```python
from build123d import *

# Parameters (mm, degrees)
PROFILE_W               = 12.7
PROFILE_H               = 22.86
PROFILE_W_2             = 6.35
PROFILE_H_2             = 12.7
BOSS_EXTRUDE1_DEPTH     = 12.7
SCREWHOLE_R             = 2.159
CUT_EXTRUDE1_DEPTH      = 7.35
CUT_EXTRUDE1_DEPTH_BACK = 7.35
SKETCH3_R               = 3.683
SKETCH3_R_2             = 2.159
CUT_EXTRUDE2_DEPTH      = 4.064
BOSS_EXTRUDE2_DEPTH     = 35.56


with BuildPart() as part:
    # Profile → Boss-Extrude1 (new body, symmetric)
    with BuildSketch(Plane.XY):
        with Locations((0, 11.43)):
            Rectangle(PROFILE_W, PROFILE_H)
        with Locations((3.175, -6.35)):
            Rectangle(PROFILE_W_2, PROFILE_H_2)
    extrude(amount=BOSS_EXTRUDE1_DEPTH, both=True)

    # ScrewHole → Cut-Extrude1 (cut, two sides)
    with BuildSketch(Plane.ZY) as cut_extrude1_sk:
        with Locations((0, -6.35)):
            Circle(SCREWHOLE_R)
    extrude(amount=CUT_EXTRUDE1_DEPTH, mode=Mode.SUBTRACT)
    extrude(cut_extrude1_sk.sketch, amount=-CUT_EXTRUDE1_DEPTH_BACK, mode=Mode.SUBTRACT)

    # Sketch3 → Cut-Extrude2 (cut)
    with BuildSketch(Plane(origin=(6.35, 0, 0), x_dir=(0, 0, -1), z_dir=(1, 0, 0))):
        with Locations((0, -6.35)):
            Circle(SKETCH3_R)
        with Locations((0, -6.35)):
            Circle(SKETCH3_R_2, mode=Mode.SUBTRACT)
    extrude(amount=-CUT_EXTRUDE2_DEPTH, mode=Mode.SUBTRACT)

    # Sketch5 → Boss-Extrude2 (add)
    with BuildSketch(Plane.XZ.offset(12.7)):
        with BuildLine():
            Line((-1.27, -57.15), (3.81, -57.15))
            Line((3.81, -57.15), (1.016473553, -32.70664359))
            ThreePointArc((1.016473553, -32.70664359), (2.103447964, -24.502378011), (6.930571429, -17.78))
            Line((6.930571429, -17.78), (6.35, -12.7))
            Line((6.35, -12.7), (0, -12.7))
            Line((0, -12.7), (-6.35, -12.7))
            Line((-6.35, -12.7), (-1.27, -57.15))
        make_face()
    extrude(amount=-BOSS_EXTRUDE2_DEPTH)


solid = part.part
```
The listing builds one solid part. Answer for the finished solid, in the listing's coordinates (mm). A direction names the side the tool comes from. Round coordinates to 2 decimals unless told otherwise and drop trailing zeros. Loops run counter-clockwise (first coordinate to the right, second up) from the corner with the lowest first, then second, coordinate; pieces in that order, holes last. Notation, with made-up numbers: (58.5, 86) - (85.5, 86) arc R14 ccw to (85.5, 107) - close; hole circle Ø3 at (-18, 65.25). An arc over 180 degrees is marked (long way). Use one line per item in the form item = value. Start each with the question number.
1. The part is cut by section D-D on y = 12. Determine the outline of the cut face in (x, z).
2. The part is cut by section A-A on z = 0. Determine the outline of the cut face in (x, y), then the cut area to 3 significant figures.
3. Given pin 1 Ø4.5 at (y, z) = (-6.35, 0) entering from +X; pin 2 Ø8 at (y, z) = (-8, 0) entering from +X; pin 3 Ø1.9 at (x, y) = (-4.5, -7.5) entering from +Z, each flat-ended and moving along its own axis, determine where each tip first touches the part or whether it passes through.
4. The part is cut by section B-B on y = -1. Determine the outline of the cut face in (x, z), then the cut area to 3 significant figures.
5. A tool of negligible diameter and unlimited length cuts with its end or side. For faces 1 (the face through (2.433, 4.831, -45.099)), 2 (the face through (2.286, -8, -2)), 3 (the face through (6.35, 5, 0)), 4 (the face through (-3, -6, -12.7)), 5 (the face through (1.127, -8.458, -0.468)), from which of +Z, -Z, +X, -X, +Y, -Y can it reach the whole face along a straight path? Write none if from no direction.
6. For a pull along Z with two mould halves and no side action, classify faces 6 (the face through (1, 5, -57.15)), 7 (the face through (0, -12.7, -22)), 8 (the face through (4.346, -9.945, 0.798)) as pulls with the +Z half, pulls with the -Z half, needs draft (parallel to the pull), parting line crosses it, or undercut.
7. The part is cut by section C-C on y = -6.35. Determine the outline of the cut face in (x, z).
8. Consider line 1 (Y direction, x = 1.65, z = 0); line 2 (Z direction, x = 0.75, y = -6.35); line 3 (X direction, y = 14, z = 6.5). Determine where each line is inside the solid, lowest interval first. Write a range as [from, to].
Geometry check:
q1.outline = (-6.35, -12.7) - (-1.27, -57.15) - (3.81, -57.15) - (1.02, -32.71) arc R17.02 cw to (6.93, -17.78) - (6.35, -12.7) - (6.35, 12.7) - (-6.35, 12.7) - close
q2.outline = (-6.35, 0) - (0, 0) - (0, -4.19) - (2.29, -4.19) - (2.29, -2.67) - (6.35, -2.67) - (6.35, 22.86) - (-6.35, 22.86) - close; (0, -12.7) - (6.35, -12.7) - (6.35, -10.03) - (2.29, -10.03) - (2.29, -8.51) - (0, -8.51) - close
q2.area = 331 mm^2
q3.pin_1 = 2.29
q3.pin_2 = 6.35
q3.pin_3 = -12.7
q4.outline = (-6.35, -12.7) - (-1.27, -57.15) - (3.81, -57.15) - (1.02, -32.71) arc R17.02 cw to (6.93, -17.78) - (6.35, -12.7) - (6.35, 12.7) - (0, 12.7) - (0, -12.7) - close
q4.area = 461 mm^2
q5.face_1 = +X, +Y, -Y
q5.face_2 = +X
q5.face_3 = +Z, +X, +Y, -Y
q5.face_4 = +Z, -X, -Y
q5.face_5 = +X, -X
q6.face_6 = pulls with the -Z half
q6.face_7 = needs draft
q6.face_8 = undercut
q7.outline = (-6.35, -12.7) - (-1.27, -57.15) - (3.81, -57.15) - (1.02, -32.71) arc R17.02 cw to (6.93, -17.78) - (6.35, -12.7) - (6.35, -3.68) - (2.29, -3.68) - (2.29, -2.16) - (0, -2.16) - (0, -12.7) - close; (0, 2.16) - (2.29, 2.16) - (2.29, 3.68) - (6.35, 3.68) - (6.35, 12.7) - (0, 12.7) - close
q8.line_1 = [-12.7, -8.51], [-4.19, 22.86]
q8.line_2 = [-57.15, -2.16], [2.16, 12.7]
q8.line_3 = [-6.35, 6.35]
